from build123d import *

# Parameters (mm, degrees)
BOSS_EXTRUDE1_DEPTH = 25.4
CUT_EXTRUDE1_REACH  = 57.721
SKETCH2_R           = 3.175
CUT_EXTRUDE2_REACH  = 53.588
SKETCH3_R           = 3.175


with BuildPart() as part:
    # Sketch1 → Boss-Extrude1 (new body)
    with BuildSketch(Plane.XY):
        Polygon((0, 0), (0, -31.75), (31.75, -31.75), (31.75, -38.1), (-6.35, -38.1), (-6.35, 0), align=None)
    extrude(amount=BOSS_EXTRUDE1_DEPTH)

    # Sketch2 → Cut-Extrude1 (cut, up to next)
    with BuildSketch(Plane(origin=(0, 0, 0), x_dir=(0, 0, -1), z_dir=(1, 0, 0)), mode=Mode.PRIVATE) as cut_extrude1_sk1:
        with Locations(Location((-12.7, -12.7, 0), (0, 0, 90))):
            Circle(SKETCH2_R)
    cut_extrude1_tool1 = extrude(cut_extrude1_sk1.sketch, amount=-CUT_EXTRUDE1_REACH, mode=Mode.PRIVATE) & part.part
    add(cut_extrude1_tool1.solids().sort_by_distance((0, -12.7, 12.7))[0], mode=Mode.SUBTRACT)

    # Sketch3 → Cut-Extrude2 (cut, up to next)
    with BuildSketch(Plane(origin=(0, -31.75, 0), x_dir=(1, 0, 0), z_dir=(0, 1, 0)), mode=Mode.PRIVATE) as cut_extrude2_sk1:
        with Locations(Location((19.05, -12.7, 0), (0, 0, 270))):
            Circle(SKETCH3_R)
    cut_extrude2_tool1 = extrude(cut_extrude2_sk1.sketch, amount=-CUT_EXTRUDE2_REACH, mode=Mode.PRIVATE) & part.part
    add(cut_extrude2_tool1.solids().sort_by_distance((19.05, -31.75, 12.7))[0], mode=Mode.SUBTRACT)


solid = part.part
Geometry: final body of the model. Coordinates: model frame, mm. A direction names the side the tool comes from. Coordinates: 2 decimals unless noted, no trailing zeros. Order: outer loops, then holes, each group sorted by start corner. A loop starts at its lowest first (then second) coordinate and runs counter-clockwise, first axis right, second up.
(1) Section query C-C (y = -12.7). Return the cut outline in (x, z) (3 decimals), plus the area to 3 significant figures.
(2) Section query D-D (x = -3). Return the cut outline in (y, z) (3 decimals).
(3) Draft query along X for faces 3 (the face through (-3.1, -11.2, 9.9)), 4 (the face through (31.75, -35, 13)), 5 (the face through (15.95, -34.88, 12.01)). Return one class per face: pulls with the +X half, pulls with the -X half, needs draft (parallel to the pull), parting line crosses it, or undercut.
(4) Access query for faces 1 (the face through (0, -16, 15)), 2 (the face through (-3, 0, 13)). Directions: +Z, -Z, +X, -X, +Y, -Y. A direction counts if a zero-diameter tool reaches every point of the face in a straight line with its end or side. Return the directions, or none.
(5) Section query B-B (x = 19.05). Return the cut outline in (y, z) (3 decimals).
(6) Material intervals for probe 1 along X at (y, z) = (-35.25, 12.7) (3 decimals); probe 2 along X at (y, z) = (-8.5, 5.75); probe 3 along Y at (x, z) = (0.5, 9.5), sorted ascending.
(7) Section query A-A (z = 12.7). Return the cut outline in (x, y) (3 decimals).
(8) First-contact query: pin 1 (10 mm diameter, centred on y = -12.7, z = 12.7, fed in from +X); pin 2 (12 mm diameter, centred on x = 5, y = -30, fed in from -Z); pin 3 (1.5 mm diameter, centred on x = 13, z = 16, fed in from +Y). Flat tips, straight axial feed; report the tip coordinate or a pass-through.
Solution:
1. outline: (-6.35, 0) - (0, 0) - (0, 9.525) - (-6.35, 9.525) - close; (-6.35, 15.875) - (0, 15.875) - (0, 25.4) - (-6.35, 25.4) - close
1. area: 121 mm2
2. outline: (-38.1, 0) - (0, 0) - (0, 25.4) - (-38.1, 25.4) - close; hole circle Ø6.35 at (-12.7, 12.7)
3. face 3: needs draft
3. face 4: pulls with the +X half
3. face 5: undercut
4. face 1: +Z, -Z, +X, +Y
4. face 2: +Z, -Z, +X, -X, +Y
5. outline: (-38.1, 0) - (-31.75, 0) - (-31.75, 9.525) - (-38.1, 9.525) - close; (-38.1, 15.875) - (-31.75, 15.875) - (-31.75, 25.4) - (-38.1, 25.4) - close
6. probe 1: x = -6.35 to 15.875, 22.225 to 31.75
6. probe 2: x = -6.35 to 0
6. probe 3: y = -38.1 to -31.75
7. outline: (-6.35, -38.1) - (15.875, -38.1) - (15.875, -31.75) - (0, -31.75) - (0, -15.875) - (-6.35, -15.875) - close; (-6.35, -9.525) - (0, -9.525) - (0, 0) - (-6.35, 0) - close; (22.225, -38.1) - (31.75, -38.1) - (31.75, -31.75) - (22.225, -31.75) - close
8. pin 1: stops at x = 0
8. pin 2: stops at z = 0
8. pin 3: stops at y = -31.75
